The figure shows three views and two pictorial views of one solid part (mm, origin at its lowest corner). Answer the questions. A direction names the side the tool comes from. Round coordinates to 2 decimals unless told otherwise and drop trailing zeros. Order: outer loops, then holes, each group sorted by start corner. A loop starts at its lowest first (then second) coordinate and runs counter-clockwise, first axis right, second up. Notation, with made-up numbers: (77.5, 80) -> (102.5, 80) arc R19 cw to (102.5, 110) -> close; hole circle Ø8 at (-23, 55.5). An arc over 180 degrees is marked (long way). Return JSON: item names as keys, results as strings. Group by question number.
(1) The part is cut by section B-B (x = 58). Determine the outline of the cut face in (y, z), plus the area to 3 significant figures.
(2) Each of these flat-tipped pins is pushed along its axis until it touches: pin 1 (2 mm diameter, centred on x = 104, y = 8, fed in from +Z); pin 2 (2 mm diameter, centred on x = 96, y = 9, fed in from -Z); pin 3 (1.5 mm diameter, centred on x = 28.5, y = 6.5, fed in from +Z). Where does it stop, or does it pass through?
(3) Which of the six approach directions +Z, -Z, +X, -X, +Y, -Y give full straight-line access (tool end or side, diameter ignored) to the marked faces 1, 2 and 3?
(4) The part is cut by section C-C (y = 4.5). Count the separate pieces of the cut face and the enclosed holes in it, plus the area to 3 significant figures.
(5) Determine the mould class of the marked faces 4, 5 and 6 for opening direction X: +X half, -X half, draft (parallel to the pull), parting line (faces both ways), or undercut.
(6) Consider line 1 (X direction, y = 9, z = 34.5); line 2 (X direction, y = 3, z = 56.8); line 3 (Z direction, x = 7.2, y = 4.5). Determine where each line is inside the solid, lowest interval first. Write a range as [from, to].
(7) The part is cut by section A-A (x = 80). Determine the outline of the cut face in (y, z).
(8) The part is cut by section D-D (z = 56.8). Determine the outline of the cut face in (x, y).
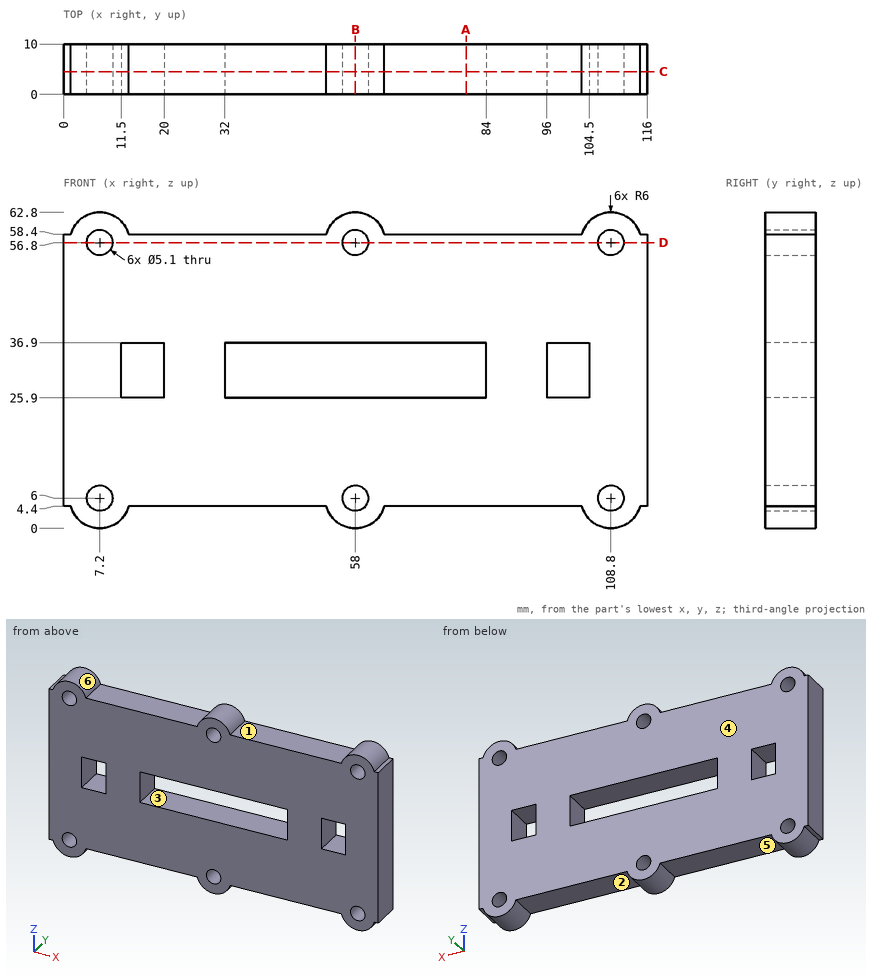
Answer below:
{
 "1": {"outline": "(0, 0) -> (10, 0) -> (10, 3.45) -> (0, 3.45) -> close; (0, 8.55) -> (10, 8.55) -> (10, 25.9) -> (0, 25.9) -> close; (0, 36.9) -> (10, 36.9) -> (10, 54.25) -> (0, 54.25) -> close; (0, 59.35) -> (10, 59.35) -> (10, 62.8) -> (0, 62.8) -> close", "area": "416 mm²"},
 "2": {"pin 1": "stops at z = 61.44", "pin 2": "stops at z = 4.4", "pin 3": "stops at z = 58.4"},
 "3": {"face 1": "+Z, +Y, -Y", "face 2": "-Z, +Y, -Y", "face 3": "+Y, -Y"},
 "4": {"separate pieces": "1", "enclosed holes": "9", "area": "5,610 mm²"},
 "5": {"face 4": "draft", "face 5": "undercut", "face 6": "undercut"},
 "6": {"line 1": "x = [0, 11.5], [20, 32], [84, 96], [104.5, 116]", "line 2": "x = [0, 4.65], [9.75, 55.45], [60.55, 106.25], [111.35, 116]", "line 3": "z = [0, 3.45], [8.55, 54.25], [59.35, 62.8]"},
 "7": {"outline": "(0, 4.4) -> (10, 4.4) -> (10, 25.9) -> (0, 25.9) -> close; (0, 36.9) -> (10, 36.9) -> (10, 58.4) -> (0, 58.4) -> close"},
 "8": {"outline": "(0, 0) -> (4.65, 0) -> (4.65, 10) -> (0, 10) -> close; (9.75, 0) -> (55.45, 0) -> (55.45, 10) -> (9.75, 10) -> close; (60.55, 0) -> (106.25, 0) -> (106.25, 10) -> (60.55, 10) -> close; (111.35, 0) -> (116, 0) -> (116, 10) -> (111.35, 10) -> close"}
}
